Source: CAD feature listing. Evaluate the final solid. Frame: model axes, mm. Face numbers are marked on the shaded views. A direction names the side the tool comes from. Round coordinates to 2 decimals unless told otherwise and drop trailing zeros. Loops run counter-clockwise (first coordinate to the right, second up) from the corner with the lowest first, then second, coordinate; pieces in that order, holes last. Notation, with made-up numbers: M -1.75,76 L 34.25,76 A27 cw 34.25,96 Z; hole C 22.25,45 d4. An arc over 180 degrees is marked long. One line per item, written item: value.
Autodesk Inventor part; units mm, degrees
ref_plane "YZ Plane" through (0, 0, 0) normal (1, 0, 0) x (0, 1, 0)
ref_plane "XZ Plane" through (0, 0, 0) normal (0, 1, 0) x (-1, 0, 0)
ref_plane "XY Plane" through (0, 0, 0) normal (0, 0, 1) x (1, 0, 0)
sketch "Sketch2" plane through (0, 0, 0) normal (0, 1, 0) x (-1, 0, 0)
  line L0 (0, 0) -> (2.54, 0)
  line L1 (2.54, 0) -> (2.54, 2.54)
  line L2 (2.54, 2.54) -> (0, 2.54)
  line L3 (0, 2.54) -> (0, 0)
  line L4 (0, 0) -> (-2.54, 0)
  line L5 (-2.54, 0) -> (-2.54, -11.43)
  line L6 (-2.54, -11.43) -> (0, -11.43)
  line L7 (0, -11.43) -> (0, 0)
  line L8 (-2.54, 0) -> (0, 0)
  line L9 (0, 0) -> (0, 2.54)
  line L10 (0, 2.54) -> (-2.54, 2.54)
  line L11 (-2.54, 2.54) -> (-2.54, 0)
  line L12 (16.51, -15.621) -> (19.05, -15.621)
  line L13 (19.05, -15.621) -> (19.05, -28.321)
  line L14 (19.05, -28.321) -> (16.51, -28.321)
  line L15 (16.51, -28.321) -> (16.51, -15.621)
  line L16 (19.05, -28.321) -> (3.81, -28.321)
  line L17 (3.81, -28.321) -> (3.81, -30.861)
  line L18 (3.81, -30.861) -> (19.05, -30.861)
  line L19 (19.05, -30.861) -> (19.05, -28.321)
  line L20 (19.05, -30.861) -> (-2.54, -30.861)
  line L21 (-2.54, -30.861) -> (-2.54, 2.54)
  line L22 (-2.54, 2.54) -> (19.05, 2.54)
  line L23 (19.05, 2.54) -> (19.05, -30.861)
  line L24 (0, 0) -> (2.54, 0)
  line L25 (2.54, 0) -> (2.54, 2.54)
  line L26 (2.54, 2.54) -> (0, 2.54)
  line L27 (0, 2.54) -> (0, 0)
  line L28 (-2.54, -11.43) -> (0, -11.43)
  line L29 (0, -11.43) -> (0, 2.54)
  line L30 (0, 2.54) -> (-2.54, 2.54)
  line L31 (-2.54, 2.54) -> (-2.54, -11.43)
  dimension "d0" = 2.54
  dimension "d1" = 2.54
  dimension "d2" = 2.54
  dimension "d3" = 11.43
  dimension "d4" = 2.54
  dimension "d5" = 12.7
  dimension "d6" = 15.24
  dimension "d7" = 2.54
  dimension "d8" = 16.51
  dimension "d9" = 28.321
extrude "Extrusion1" add sketch "Sketch2" along normal blind 10.16 contours L3 L2 L1 L0 | L4 L11 L10 L3 | L7 L6 L5 L4 | L13 L14 L15 L12 | L17 L16 L14 L19 L18
extrude "Extrusion2" add sketch "Sketch2" against normal blind 1.5875
sketch "Sketch4" plane through (0, 0, 0) normal (0, 1, 0) x (1, 0, 0)
  circle A0 centre (-12.7, 3.9624) radius 1.5875
  circle A1 centre (-12.7, 24.3586) radius 1.5875
  line L0 (-19.05, 15.621) -> (-19.05, -2.54)
  line L1 (-19.05, -2.54) -> (-2.54, -2.54)
  line L2 (2.54, 30.861) -> (-3.81, 30.861)
  point P0 (0, 0)
  dimension "d14" = 3.175
  dimension "d15" = 3.175
  dimension "d16" = 6.35
  dimension "d17" = 6.35
  dimension "d23" = 20.3962
  dimension "d24" = 6.5024
  dimension "d25" = 33.401
extrude "Extrusion3" cut sketch "Sketch4" against normal blind 1.5875
fillet "Fillet1" radius 3.175 4 edges at (2.54, -0.7937, -30.861) (2.54, 4.2862, 2.54) (-19.05, -0.7937, 2.54) (-19.05, 4.2863, -30.861)
chamfer "Chamfer1" distance 1.27 angle 45 2 edges at (-14.2875, 0, -24.3586) (-14.2875, 0, -3.9624)
equation "\"d24\" = -0.5 * d23 + 0.5 * d25"
properties part number "limitSwitchHolder2" material "ABS Plastic"
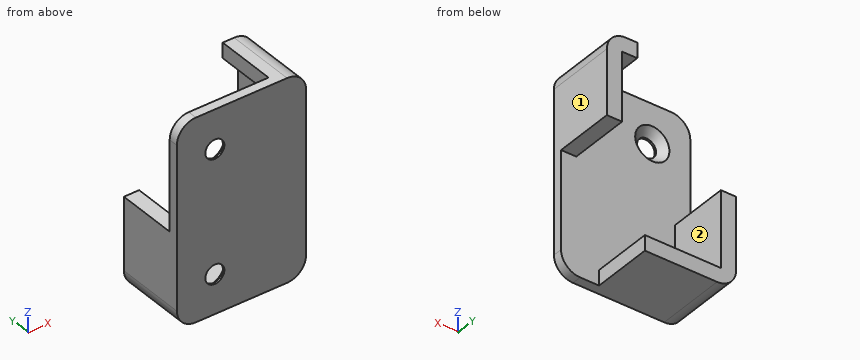
1. Section query D-D (x = -8). Return the cut outline in (y, z), and give its area (3 significant figures).
Report:
outline: M -1.59,-30.86 L 10.16,-30.86 L 10.16,-28.32 L 0,-28.32 L 0,2.54 L -1.59,2.54 Z
area: 78.8 mm2
2. Pin query (flat end, axial travel): pin 1 (1 mm diameter, centred on x = -11.5, z = -27, fed in from +Y); pin 2 (5 mm diameter, centred on x = -12.7, z = -3.96, fed in from +Y); pin 3 (0.8 mm diameter, centred on x = 2, y = 5.5, fed in from -Z). Return the tip coordinate at first contact, or that it passes through.
Report:
pin 1: stops at y = 0
pin 2: stops at y = -0.36
pin 3: stops at z = -11.43
3. Reachability of the marked faces 1 and 2 from +Z, -Z, +X, -X, +Y, -Y: full face, straight path, thin tool, end or side. Return the list, or none.
Report:
face 1: +Z, -Z, +X, +Y, -Y
face 2: +Z, +X, +Y
4. Section query A-A (y = 9.5). Return the cut outline in (x, z) (3 decimals).
Report:
outline: M -19.05,-27.686 A3.175 ccw -15.875,-30.861 L -3.81,-30.861 L -3.81,-28.321 L -16.51,-28.321 L -16.51,-15.621 L -19.05,-15.621 Z; M -2.54,0 L 0,0 L 0,-11.43 L 2.54,-11.43 L 2.54,-0.635 A3.175 ccw -0.635,2.54 L -2.54,2.54 Z
5. Section query B-B (x = -12.7). Return the cut outline in (y, z).
Report:
outline: M -1.59,-30.86 L 10.16,-30.86 L 10.16,-28.32 L 0,-28.32 L 0,-27.22 L -1.27,-25.95 L -1.59,-25.95 Z; M -1.59,-22.77 L -1.27,-22.77 L 0,-21.5 L 0,-6.82 L -1.27,-5.55 L -1.59,-5.55 Z; M -1.59,-2.37 L -1.27,-2.37 L 0,-1.1 L 0,2.54 L -1.59,2.54 Z
6. Section query C-C (z = -16). Return the cut outline in (x, y), and give its area (3 significant figures).
Report:
outline: M -19.05,-1.59 L 2.54,-1.59 L 2.54,0 L -16.51,0 L -16.51,10.16 L -19.05,10.16 Z
area: 60.1 mm2
7. Ray query, line 1 (Z direction, x = -12.7, y = -1.45); line 2 (Y direction, x = -5, z = -22); line 3 (Z direction, x = -14, y = 6.5). Return the intervals inside material, ascending. Write a range as [from, to].
Report:
line 1: z = [-30.86, -25.95], [-22.77, -5.55], [-2.37, 2.54]
line 2: y = [-1.59, 0]
line 3: z = [-30.86, -28.32]
